```python
from build123d import *

# Parameters (mm, degrees)
F0_W     = 1219.2
F0_H     = 355.6
F1_DEPTH = 36.83
F2_W     = 39.37
F2_H     = 177.8
F3_DEPTH = 36.83


with BuildPart() as f1:
    # F0 (on Top) → F1 (new body)
    with BuildSketch(Plane.XY):
        Rectangle(F0_W, F0_H)
    extrude(amount=F1_DEPTH)

    # F2 (on face) → F3 (cut, through all)
    with BuildSketch(Plane.XY.offset(36.83)):
        with Locations((-527.685, 88.9)):
            Rectangle(F2_W, F2_H)
        with Locations((527.685, 88.9)):
            Rectangle(F2_W, F2_H)
    extrude(amount=-F3_DEPTH, mode=Mode.SUBTRACT)


solid = f1.part
```
Input: part model. Units: mm. Frame: model coordinates. A direction names the side the tool comes from. Coordinates: 2 decimals unless noted, no trailing zeros. Write each loop counter-clockwise with the first axis right and the second up, starting at its lowest first coordinate (ties: lowest second). Pieces come first, ordered by that corner, then holes. Notation, with made-up numbers: (-4, -2) -> (2, -2) arc R25 cw to (2, 19) -> close; hole circle Ø5 at (7.5, 82.25). An arc over 180 degrees is marked (long way). Write each question's results on one line, items separated by ' | '.
Item 1: Pin query (flat end, axial travel): pin 1 Ø1 at (x, y) = (81, -130) entering from -Z. Return the tip coordinate at first contact, or that it passes through.
Conclusion:
pin 1: stops at z = 0
Item 2: Set-up query: faces 1 (the flat face through (-528, 0, 19)), 2 (the flat face through (609.6, -2, 18)). Return all of +Z, -Z, +X, -X, +Y, -Y with unobstructed straight access to the full face (end or side cutting, diameter ignored); none if empty.
Conclusion:
face 1: +Z, -Z, +Y | face 2: +Z, -Z, +X, +Y, -Y
Item 3: Section query B-B on z = 18.5. Return loops of the section in (x, y), plus the area to 3 significant figures.
Conclusion:
outline: (-609.6, -177.8) -> (609.6, -177.8) -> (609.6, 177.8) -> (547.37, 177.8) -> (547.37, 0) -> (508, 0) -> (508, 177.8) -> (-508, 177.8) -> (-508, 0) -> (-547.37, 0) -> (-547.37, 177.8) -> (-609.6, 177.8) -> close | area: 420,000 mm^2
Item 4: Material intervals for probe 1 along X at (y, z) = (153, 9); probe 2 along Y at (x, z) = (531, 25.5), sorted ascending.
Conclusion:
probe 1: x = -609.6 to -547.37, -508 to 508, 547.37 to 609.6 | probe 2: y = -177.8 to 0
Item 5: Mould query, pull axis X, two halves, no side actions, for faces 3 (the flat face through (-609.6, -2, 18)), 4 (the flat face through (547.37, 88, 19)), 5 (the flat face through (-7, 177.8, 18)). Classes: +X half, -X half, draft (parallel to the pull), parting line (faces both ways), or undercut.
Conclusion:
face 3: -X half | face 4: undercut | face 5: draft
Item 6: Section query A-A on y = 152.5. Return loops of the section in (x, z), plus the area to 3 significant figures.
Conclusion:
outline: (-609.6, 0) -> (-547.37, 0) -> (-547.37, 36.83) -> (-609.6, 36.83) -> close; (-508, 0) -> (508, 0) -> (508, 36.83) -> (-508, 36.83) -> close; (547.37, 0) -> (609.6, 0) -> (609.6, 36.83) -> (547.37, 36.83) -> close | area: 42,000 mm^2
